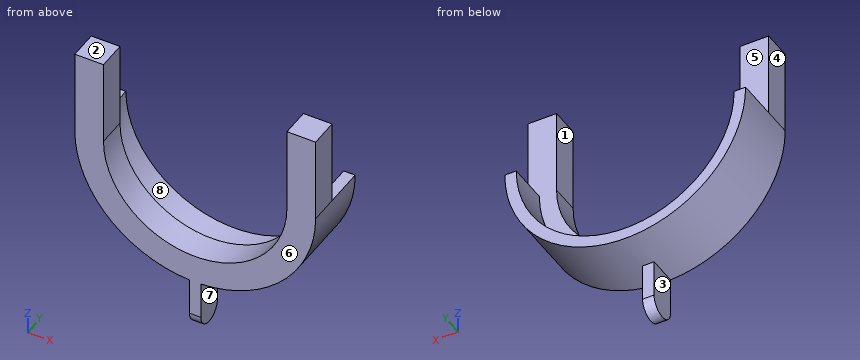
```python
from build123d import *

# Parameters (mm, degrees)
EXTRUDE_1_DEPTH     = 10
EXTRUDE_2_DEPTH     = 24
SKETCH_3_W          = 4
SKETCH_3_H          = 24
SKETCH_3_W_2        = 10
SKETCH_3_H_2        = 30
EXTRUDE_3_DEPTH     = 10
CUT_EXTRUDE_1_DEPTH = 10


with BuildPart() as part:
    # 草图1 → 凸台-拉伸1 (new body)
    with BuildSketch(Plane(origin=(0, 0, 0), x_dir=(1, 0, 0), z_dir=(0, 1, 0))):
        with BuildLine():
            Line((-38, 0), (-32, 0))
            ThreePointArc((-32, 0), (0, 32), (32, 0))
            Line((32, 0), (38, 0))
            ThreePointArc((38, 0), (0, 38), (-38, 0))
        make_face()
    extrude(amount=EXTRUDE_1_DEPTH)

    # 草图2 → 凸台-拉伸2 (add)
    with BuildSketch(Plane.XZ):
        with BuildLine():
            Line((-38, 0), (-42, 0))
            ThreePointArc((-42, 0), (0, -42), (42, 0))
            Line((42, 0), (38, 0))
            ThreePointArc((38, 0), (0, -38), (-38, 0))
        make_face()
    extrude(amount=-EXTRUDE_2_DEPTH)

    # 草图3 → 凸台-拉伸3 (add)
    with BuildSketch(Plane.XZ):
        with Locations((0, -48)):
            Rectangle(SKETCH_3_W, SKETCH_3_H)
        with Locations((-37, 15)):
            Rectangle(SKETCH_3_W_2, SKETCH_3_H_2)
        with Locations((37, 15)):
            Rectangle(SKETCH_3_W_2, SKETCH_3_H_2)
    extrude(amount=-EXTRUDE_3_DEPTH)

    # 草图4 → 切除-拉伸1 (cut)
    with BuildSketch(Plane.ZY.offset(2)):
        with BuildLine():
            Line((-55, 10), (-63.230439801, 10))
            Line((-63.230439801, 10), (-63.230439801, 0))
            Line((-63.230439801, 0), (-55, 0))
            ThreePointArc((-55, 0), (-60, 5), (-55, 10))
        make_face()
    extrude(amount=-CUT_EXTRUDE_1_DEPTH, mode=Mode.SUBTRACT)


solid = part.part
```
Build history of the part. All positions in model axes, mm. Face numbers are marked on the shaded views. A direction names the side the tool comes from. Round coordinates to 2 decimals unless told otherwise and drop trailing zeros. Order: outer loops, then holes, each group sorted by start corner. A loop starts at its lowest first (then second) coordinate and runs counter-clockwise, first axis right, second up. Notation, with made-up numbers: (-22, 74) - (27, 74) arc R24 ccw to (27, 97) - close; hole circle Ø10 at (56.25, -6.5). An arc over 180 degrees is marked (long way). Use a Markdown table: item, result.
1) Saw through at B-B on x = 0. Write the cut outline in (y, z).
Recorded:
| item | result |
|---|---|
| outline | (0, -55) arc R5 ccw to (10, -55) - (10, -42) - (24, -42) - (24, -38) - (10, -38) - (10, -32) - (0, -32) - close |
2) Pull direction X, two halves, no side cores. Call the marked faces 6, 7 and 8: pulls with the +X half, pulls with the -X half, needs draft (parallel to the pull), parting line crosses it, or undercut.
Recorded:
| item | result |
|---|---|
| face 6 | needs draft |
| face 7 | pulls with the +X half |
| face 8 | undercut |
3) Flat gauge pins, fed straight in: pin 1 Ø2 at (x, z) = (29.5, 20.5) entering from +Y; pin 2 Ø2 at (x, y) = (40, 16) entering from +Z; pin 3 Ø2 at (x, z) = (0.5, -50.5) entering from +Y; pin 4 Ø4 at (x, y) = (6, 4.5) entering from -Z. Where does each tip first touch, or does it go through?
Recorded:
| item | result |
|---|---|
| pin 1 | passes through |
| pin 2 | stops at z = 0 |
| pin 3 | stops at y = 10 |
| pin 4 | stops at z = -41.81 |
4) Saw through at C-C on z = -24.5. Write the cut outline in (x, y).
Recorded:
| item | result |
|---|---|
| outline | (-34.11, 0) - (-20.59, 0) - (-20.59, 10) - (-29.05, 10) - (-29.05, 24) - (-34.11, 24) - close; (20.59, 0) - (34.11, 0) - (34.11, 24) - (29.05, 24) - (29.05, 10) - (20.59, 10) - close |
5) Wall check: L1, parallel to X at y = 7.5, z = 6; L2, parallel to X at y = 19.75, z = -0.5; L3, parallel to Y at x = 33, z = 11. Give the ranges that are in metal, low to high.
Recorded:
| item | result |
|---|---|
| L1 | x = -42 to -32, 32 to 42 |
| L2 | x = -42 to -38, 38 to 42 |
| L3 | y = 0 to 10 |
6) Saw through at A-A on y = 5. Write the cut outline in (x, z), and give its area (3 significant figures).
Recorded:
| item | result |
|---|---|
| outline | (-42, 0) arc R42 ccw to (-2, -41.95) - (-2, -60) - (2, -60) - (2, -41.95) arc R42 ccw to (42, 0) - (42, 30) - (32, 30) - (32, 0) arc R32 cw to (-32, 0) - (-32, 30) - (-42, 30) - close |
| area | 1,830 mm² |
7) Tool access for the marked faces 1, 2, 3, 4 and 5: list every direction of +Z, -Z, +X, -X, +Y, -Y with a clear straight run to the whole face (end or side of a thin tool).
Recorded:
| item | result |
|---|---|
| face 1 | +Z, +Y, -Y |
| face 2 | +Z, +X, -X, +Y, -Y |
| face 3 | -Z, -X, +Y, -Y |
| face 4 | +Z, -Z, -X, +Y, -Y |
| face 5 | +Z, +Y |
8) Saw through at D-D on z = -13. Write the cut outline in (x, y), and give its area (3 significant figures).
Recorded:
| item | result |
|---|---|
| outline | (-39.94, 0) - (-29.24, 0) - (-29.24, 10) - (-35.71, 10) - (-35.71, 24) - (-39.94, 24) - close; (29.24, 0) - (39.94, 0) - (39.94, 24) - (35.71, 24) - (35.71, 10) - (29.24, 10) - close |
| area | 332 mm² |
